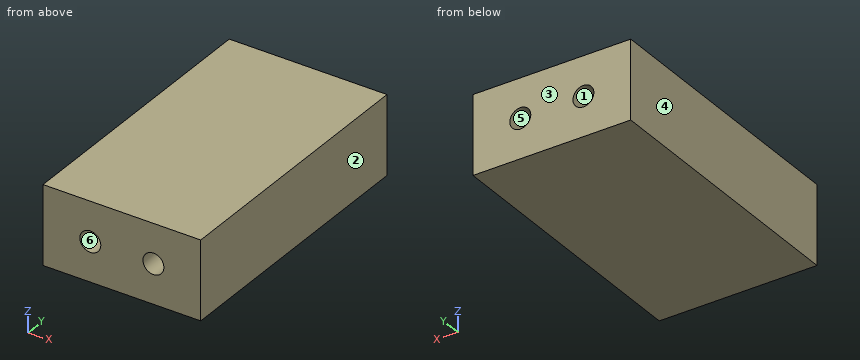
Autodesk Inventor part; units mm, degrees
ref_plane "YZ Plane" through (0, 0, 0) normal (1, 0, 0) x (0, 1, 0)
ref_plane "XZ Plane" through (0, 0, 0) normal (0, 1, 0) x (-1, 0, 0)
ref_plane "XY Plane" through (0, 0, 0) normal (0, 0, 1) x (1, 0, 0)
sketch "Sketch1" plane through (0, 0, 0) normal (0, 1, 0) x (-1, 0, 0)
  line L0 (0, 0) -> (-31.75, 0)
  line L1 (-31.75, 0) -> (-31.75, -15.875)
  line L2 (-31.75, -15.875) -> (0, -15.875)
  line L3 (0, -15.875) -> (0, 0)
  dimension "d0" = 15.875
  dimension "d1" = 31.75
extrude "Extrusion1" add sketch "Sketch1" along normal blind 55.88
sketch "Sketch2" plane through (0, 55.88, 0) normal (0, 1, 0) x (1, 0, 0)
  line L0 (0, 15.875) -> (0, 0)
  line L1 (31.75, 0) -> (31.75, 15.875)
  line L2 (31.75, 15.875) -> (0, 15.875)
  line L3 (0, 0) -> (31.75, 0)
  point P0 (9.525, 7.9375)
  point P1 (22.225, 7.9375)
  dimension "d5" = 12.7
  dimension "d25" = 15.875
  dimension "d26" = 7.9375
  dimension "d27" = 9.525
hole "Hole1" at (9.525, 55.88, -7.9375) at (22.225, 55.88, -7.9375) direction (0, -1, 0) diameter 4.2164 depth 6.35 tip angle 118
sketch "Sketch3" plane through (0, 0, 0) normal (0, -1, 0) x (1, 0, 0)
  circle A0 centre (9.525, -7.9375) radius 2.1082
  circle A1 centre (22.225, -7.9375) radius 2.1082
  point P0 (0, 0)
hole "Hole2" at (9.525, 0, -7.9375) at (22.225, 0, -7.9375) direction (0, 1, 0) diameter 4.2164 depth 6.35 tip angle 118
properties part number "Garalite Support"
Build history of the part. All positions in model axes, mm. Face numbers are marked on the shaded views. A direction names the side the tool comes from. Give positions to 0.01 mm unless a question says otherwise; leave off trailing zeros.
1) 3-axis set-ups, long thin cutter, end or side, ignore diameter. For the marked faces 4, 5 and 6: which of +Z, -Z, +X, -X, +Y, -Y reach the whole face in a straight line?
Values follow:
face 4: +Z, -Z, -X, +Y, -Y
face 5: +Y
face 6: -Y
2) Band-saw the part on A-A on y = 4. State how many separate pieces and enclosed holes the cut face has, then the cut area to 3 significant figures.
Values follow:
separate pieces: 1
enclosed holes: 2
area: 476 mm2
3) Probe line 1 along Z through (x, y) = (11, 3) (3 decimals). List the from-to ranges inside material, lowest first.
Values follow:
line 1: z = -15.875 to -9.444, -6.431 to 0
4) Two-plate mould, pull along X, no slides. Class the marked faces 1, 2 and 3: released by +X, released by -X, zero draft, split by the parting line, or undercut.
Values follow:
face 1: undercut
face 2: released by +X
face 3: zero draft
